Can you work these out from the drawing? Everything is in mm from the part's minimum corner. A direction names the side the tool comes from. Round coordinates to 2 decimals unless told otherwise and drop trailing zeros. Order: outer loops, then holes, each group sorted by start corner. A loop starts at its lowest first (then second) coordinate and runs counter-clockwise, first axis right, second up. Notation, with made-up numbers: (48.5, -26) -> (83.5, -26) arc R23 ccw to (83.5, -12) -> close; hole circle Ø9 at (-15.75, -31.5). An arc over 180 degrees is marked (long way). One line per item, written item: value.
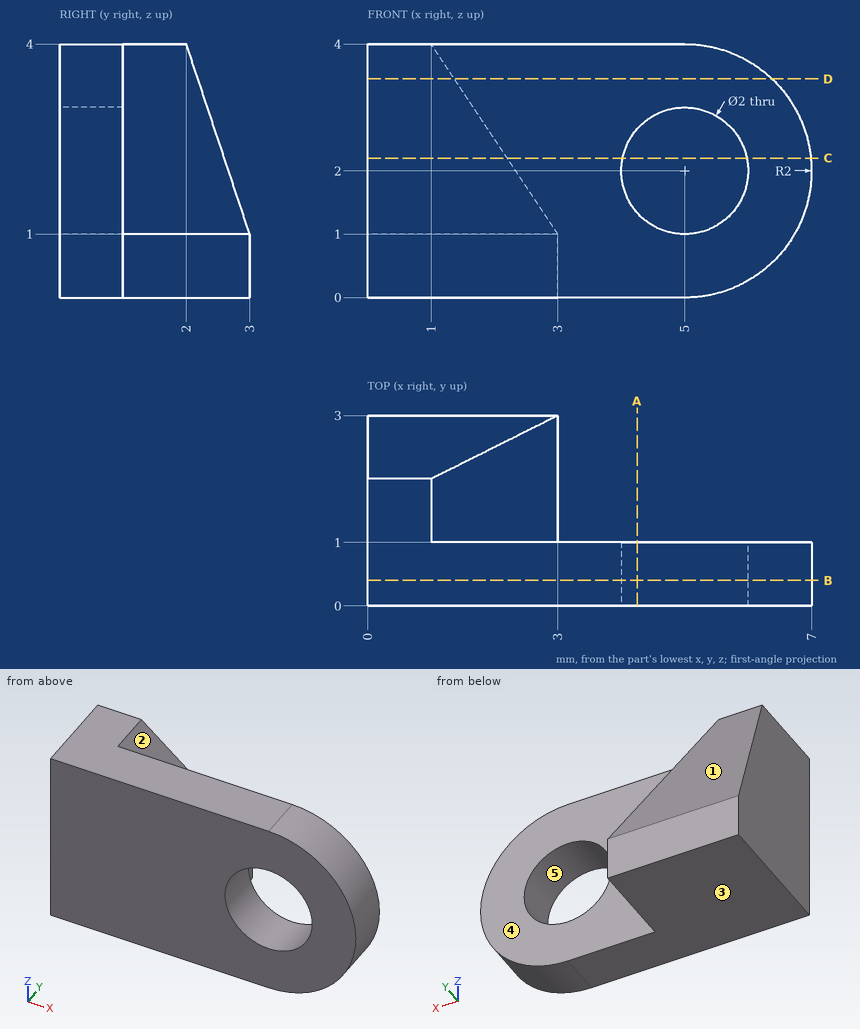
Q1. I want a section at A-A on x = 4.25. List the corners of the cut face in (y, z) for me.
Answers below:
outline: (0, 0) -> (1, 0) -> (1, 1.34) -> (0, 1.34) -> close; (0, 2.66) -> (1, 2.66) -> (1, 4) -> (0, 4) -> close
Q2. I want a section at C-C on z = 2.2. List the corners of the cut face in (x, y) for me.
Answers below:
outline: (0, 0) -> (4.02, 0) -> (4.02, 1) -> (2.2, 1) -> (2.2, 2.6) -> (0, 2.6) -> close; (5.98, 0) -> (6.99, 0) -> (6.99, 1) -> (5.98, 1) -> close
Q3. Please list where these lines run through material, in increasing order: line 1 along Z through (x, y) = (5, 0.55); line 2 along X through (y, z) = (1.95, 0.9); line 3 along Y through (x, z) = (3.5, 1.05).
Answers below:
line 1: 0 to 1, 3 to 4
line 2: 0 to 3
line 3: 0 to 1
Q4. Will these pins go through, and if not, where does the flat tip stop? pin 1 Ø1.2 at (x, z) = (2.5, 3) entering from +Y; pin 2 Ø1.6 at (x, z) = (5, 2) entering from +Y; pin 3 Ø0.5 at (y, z) = (2.5, 0.5) entering from +X.
Answers below:
pin 1: y = 1
pin 2: through
pin 3: x = 3
Q5. On a 3-axis mill with a long thin cutter (end or side, diameter ignored), from which of +Z, -Z, +X, -X, +Y, -Y can I reach the whole of each face in a straight line? I mean the marked faces 1 and 2. Say none if no direction works.
Answers below:
face 1: +Z, +X, -X, +Y
face 2: +Z, +X, +Y
Q6. I want a section at D-D on z = 3.45. List the corners of the cut face in (x, y) for me.
Answers below:
outline: (0, 0) -> (6.38, 0) -> (6.38, 1) -> (1.37, 1) -> (1.37, 2.18) -> (0, 2.18) -> close
Q7. I want a section at B-B on y = 0.4. List the corners of the cut face in (x, z) for me.
Answers below:
outline: (0, 0) -> (5, 0) arc R2 ccw to (5, 4) -> (0, 4) -> close; hole circle Ø2 at (5, 2)
Q8. We'd pull the mould along Z, two halves only. Please class the marked faces 3, 4 and 5: released by +Z, released by -Z, zero draft, split by the parting line, or undercut.
Answers below:
face 3: released by -Z
face 4: zero draft
face 5: undercut
